```python
from build123d import *

# Parameters (mm, degrees)
SKETCH2_R           = 110
SKETCH2_R_2         = 11.25
SKETCH2_R_3         = 7.5
BOSS_EXTRUDE1_DEPTH = 5
BOSS_EXTRUDE2_START = 3
SKETCH1_R           = 110
SKETCH1_R_2         = 7.5
BOSS_EXTRUDE2_DEPTH = 3


with BuildPart() as part:
    # Sketch2 → Boss-Extrude1 (new body)
    with BuildSketch(Plane(origin=(0, 0, 0), x_dir=(1, 0, 0), z_dir=(0, 1, 0))):
        with Locations(Location((0, 0, 0), (0, 0, 270))):
            Circle(SKETCH2_R)
        with Locations(Location((0, 45, 0), (0, 0, 270))):
            Circle(SKETCH2_R_2, mode=Mode.SUBTRACT)
        with Locations(Location((22.5, 38.97114317, 0), (0, 0, 270))):
            Circle(SKETCH2_R_2, mode=Mode.SUBTRACT)
        with Locations(Location((38.97114317, 22.5, 0), (0, 0, 270))):
            Circle(SKETCH2_R_2, mode=Mode.SUBTRACT)
        with Locations(Location((45, 0, 0), (0, 0, 270))):
            Circle(SKETCH2_R_2, mode=Mode.SUBTRACT)
        with Locations(Location((38.97114317, -22.5, 0), (0, 0, 270))):
            Circle(SKETCH2_R_2, mode=Mode.SUBTRACT)
        with Locations(Location((22.5, -38.97114317, 0), (0, 0, 270))):
            Circle(SKETCH2_R_2, mode=Mode.SUBTRACT)
        with Locations(Location((0, -45, 0), (0, 0, 270))):
            Circle(SKETCH2_R_2, mode=Mode.SUBTRACT)
        with Locations(Location((-22.5, -38.97114317, 0), (0, 0, 270))):
            Circle(SKETCH2_R_2, mode=Mode.SUBTRACT)
        with Locations(Location((-38.97114317, -22.5, 0), (0, 0, 270))):
            Circle(SKETCH2_R_2, mode=Mode.SUBTRACT)
        with Locations(Location((-45, 0, 0), (0, 0, 270))):
            Circle(SKETCH2_R_2, mode=Mode.SUBTRACT)
        with Locations(Location((0, 0, 0), (0, 0, 270))):
            Circle(SKETCH2_R_3, mode=Mode.SUBTRACT)
        with Locations(Location((-38.97114317, 22.5, 0), (0, 0, 270))):
            Circle(SKETCH2_R_2, mode=Mode.SUBTRACT)
        with Locations(Location((-22.5, 38.97114317, 0), (0, 0, 270))):
            Circle(SKETCH2_R_2, mode=Mode.SUBTRACT)
        with Locations(Location((0, 90, 0), (0, 0, 270))):
            Circle(SKETCH2_R_2, mode=Mode.SUBTRACT)
        with Locations(Location((27.811529494, 85.595086467, 0), (0, 0, 270))):
            Circle(SKETCH2_R_2, mode=Mode.SUBTRACT)
        with Locations(Location((52.900672706, 72.811529494, 0), (0, 0, 270))):
            Circle(SKETCH2_R_2, mode=Mode.SUBTRACT)
        with Locations(Location((72.811529494, 52.900672706, 0), (0, 0, 270))):
            Circle(SKETCH2_R_2, mode=Mode.SUBTRACT)
        with Locations(Location((85.595086467, 27.811529494, 0), (0, 0, 270))):
            Circle(SKETCH2_R_2, mode=Mode.SUBTRACT)
        with Locations(Location((90, 0, 0), (0, 0, 270))):
            Circle(SKETCH2_R_2, mode=Mode.SUBTRACT)
        with Locations(Location((85.595086467, -27.811529494, 0), (0, 0, 270))):
            Circle(SKETCH2_R_2, mode=Mode.SUBTRACT)
        with Locations(Location((72.811529494, -52.900672706, 0), (0, 0, 270))):
            Circle(SKETCH2_R_2, mode=Mode.SUBTRACT)
        with Locations(Location((52.900672706, -72.811529494, 0), (0, 0, 270))):
            Circle(SKETCH2_R_2, mode=Mode.SUBTRACT)
        with Locations(Location((27.811529494, -85.595086467, 0), (0, 0, 270))):
            Circle(SKETCH2_R_2, mode=Mode.SUBTRACT)
        with Locations(Location((0, -90, 0), (0, 0, 270))):
            Circle(SKETCH2_R_2, mode=Mode.SUBTRACT)
        with Locations(Location((-27.811529494, -85.595086467, 0), (0, 0, 270))):
            Circle(SKETCH2_R_2, mode=Mode.SUBTRACT)
        with Locations(Location((-52.900672706, -72.811529494, 0), (0, 0, 270))):
            Circle(SKETCH2_R_2, mode=Mode.SUBTRACT)
        with Locations(Location((-72.811529494, -52.900672706, 0), (0, 0, 270))):
            Circle(SKETCH2_R_2, mode=Mode.SUBTRACT)
        with Locations(Location((-85.595086467, -27.811529494, 0), (0, 0, 270))):
            Circle(SKETCH2_R_2, mode=Mode.SUBTRACT)
        with Locations(Location((-90, 0, 0), (0, 0, 270))):
            Circle(SKETCH2_R_2, mode=Mode.SUBTRACT)
        with Locations(Location((-85.595086467, 27.811529494, 0), (0, 0, 270))):
            Circle(SKETCH2_R_2, mode=Mode.SUBTRACT)
        with Locations(Location((-72.811529494, 52.900672706, 0), (0, 0, 270))):
            Circle(SKETCH2_R_2, mode=Mode.SUBTRACT)
        with Locations(Location((-52.900672706, 72.811529494, 0), (0, 0, 270))):
            Circle(SKETCH2_R_2, mode=Mode.SUBTRACT)
        with Locations(Location((-27.811529494, 85.595086467, 0), (0, 0, 270))):
            Circle(SKETCH2_R_2, mode=Mode.SUBTRACT)
    extrude(amount=-BOSS_EXTRUDE1_DEPTH)

    # Sketch1 → Boss-Extrude2 (add)
    with BuildSketch(Plane(origin=(0, 0, 0), x_dir=(1, 0, 0), z_dir=(0, 1, 0)).offset(BOSS_EXTRUDE2_START)):
        with Locations(Location((0, 0, 0), (0, 0, 270))):
            Circle(SKETCH1_R)
        with Locations(Location((0, 0, 0), (0, 0, 270))):
            Circle(SKETCH1_R_2, mode=Mode.SUBTRACT)
    extrude(amount=-BOSS_EXTRUDE2_DEPTH)


solid = part.part
```
Source: CAD feature listing. Evaluate the final solid. Frame: model axes, mm. Give positions to 0.01 mm unless a question says otherwise; leave off trailing zeros. Loops run counter-clockwise (first coordinate to the right, second up) from the corner with the lowest first, then second, coordinate; pieces in that order, holes last. Notation, with made-up numbers: (36, 3.5) -> (91, 3.5) arc R21 ccw to (91, 11.5) -> close; hole circle Ø10 at (35, 82). An arc over 180 degrees is marked (long way). Put each result on its own line as item: value. Start each with the question number.
1) Cut plane D-D (x = 90). Return loops of the section in (y, z).
2) Material intervals for probe 1 along X at (y, z) = (-3.75, -43); probe 2 along X at (y, z) = (-3.1, 45); probe 3 along X at (y, z) = (-1.5, 91), sorted ascending.
3) Cut plane C-C (z = 22.5). Return loops of the section in (x, y).
4) Draft query along X for faces 1 (the face through (-97.59, -0.94, 50.76)), 2 (the face through (-79.657, -2.465, 43.973)). Return one class per face: released by +X, released by -X, zero draft, split by the parting line, or undercut.
5) Cut plane A-A (x = 0). Return loops of the section in (y, z), then the cut area to 3 significant figures.
6) Contact query for flat-ended pins moving along their axis: P1, Ø1, axis at x = -4, y = -2, coming from the -Z side; P2, Ø18, axis at x = -0.5, z = -44, coming from the -Y side. Output: stop coordinate, or through.
7) Cut plane B-B (y = -1.25). State how many separate pieces and enclosed holes the cut face has, then the cut area to 3 significant figures.
Results are:
1. outline: (-5, -63.25) -> (3, -63.25) -> (3, 63.25) -> (-5, 63.25) -> (-5, 38.16) -> (0, 38.16) -> (0, 17.46) -> (-5, 17.46) -> (-5, 11.25) -> (0, 11.25) -> (0, -11.25) -> (-5, -11.25) -> (-5, -17.46) -> (0, -17.46) -> (0, -38.16) -> (-5, -38.16) -> close
2. probe 1: x = -101.25 to -78.15, -67.47 to -33, -12 to -11.07, 11.07 to 12, 33 to 67.47, 78.15 to 101.25
2. probe 2: x = -100.37 to -80.82, -64.8 to -32, -13 to -11.25, 11.25 to 13, 32 to 64.8, 80.82 to 100.37
2. probe 3: x = -61.8 to -37.68, -17.94 to -11.21, 11.21 to 17.94, 37.68 to 61.8
3. outline: (-107.67, -5) -> (-95.51, -5) -> (-95.51, 0) -> (-75.68, 0) -> (-75.68, -5) -> (-50.22, -5) -> (-50.22, 0) -> (-27.72, 0) -> (-27.72, -5) -> (27.72, -5) -> (27.72, 0) -> (50.22, 0) -> (50.22, -5) -> (75.68, -5) -> (75.68, 0) -> (95.51, 0) -> (95.51, -5) -> (107.67, -5) -> (107.67, 3) -> (-107.67, 3) -> close
4. face 1: split by the parting line
4. face 2: undercut
5. outline: (-5, -110) -> (3, -110) -> (3, -7.5) -> (-5, -7.5) -> (-5, -33.75) -> (0, -33.75) -> (0, -56.25) -> (-5, -56.25) -> (-5, -78.75) -> (0, -78.75) -> (0, -101.25) -> (-5, -101.25) -> close; (-5, 7.5) -> (3, 7.5) -> (3, 110) -> (-5, 110) -> (-5, 101.25) -> (0, 101.25) -> (0, 78.75) -> (-5, 78.75) -> (-5, 56.25) -> (0, 56.25) -> (0, 33.75) -> (-5, 33.75) -> close
5. area: 1,190 mm2
6. P1: stops at z = -109.94
6. P2: stops at y = 0
7. separate pieces: 1
7. enclosed holes: 33
7. area: 25,100 mm2
